```python
from build123d import *

# Parameters (mm, degrees)
F1_DEPTH  = 60
F3_DEPTH  = 10
F5_DEPTH  = 10
F6_R      = 1.5
F7_R      = 1.5
F8_R      = 1.5
F9_R      = 1.5
F10_DEPTH = 10
F11_R     = 3.5
F12_DEPTH = 4
F13_R     = 1.5
F14_DEPTH = 6


# Not quite as in the source:
# - a feature names something its author has since deleted; it is built from what else it names


with BuildPart() as f1:
    # F0 (on Front) → F1 (new body)
    with BuildSketch(Plane.XZ):
        Polygon((-40, 60), (-40, 0), (40, 0), (40, 60), (30, 60), (30, 20), (12, 20), (12, 10), (-12, 10), (-12, 20), (-30, 20), (-30, 60), align=None)
    extrude(amount=F1_DEPTH)

    # F2 (on face) → F3 (cut, through all)
    with BuildSketch(Plane.YZ.offset(40)):
        with BuildLine():
            ThreePointArc((-33.5355339059, 48.5355339059), (-30, 47.0710678119), (-26.4644660941, 48.5355339059))
            Line((-26.4644660941, 48.5355339059), (-15, 60))
            Line((-15, 60), (-45, 60))
            Line((-45, 60), (-33.5355339059, 48.5355339059))
        make_face()
    extrude(amount=-F3_DEPTH, mode=Mode.SUBTRACT)

    # F4 (on face) → F5 (cut, through all)
    with BuildSketch(Plane(origin=(-40, 0, 0), x_dir=(0, -1, 0), z_dir=(-1, 0, 0))):
        with BuildLine():
            Line((37.5, 60), (22.5, 60))
            Line((22.5, 60), (26.4644660941, 56.0355339059))
            ThreePointArc((26.4644660941, 56.0355339059), (30, 54.5710678119), (33.5355339059, 56.0355339059))
            Line((33.5355339059, 56.0355339059), (37.5, 60))
        make_face()
    extrude(amount=-F5_DEPTH, mode=Mode.SUBTRACT)

    # F6 (on face) + F7 (on face) + F8 (on face) + F9 (on face) → F10 (cut)
    with BuildSketch(Plane.XY.offset(60)):
        with Locations((-35, -7.5)):
            Circle(F6_R)
    with BuildSketch(Plane.XY.offset(60)):
        with Locations((-35, -52.5)):
            Circle(F7_R)
    with BuildSketch(Plane.XY.offset(60)):
        with Locations((35, -7.5)):
            Circle(F8_R)
    with BuildSketch(Plane.XY.offset(60)):
        with Locations((35, -52.5)):
            Circle(F9_R)
    extrude(amount=-F10_DEPTH, mode=Mode.SUBTRACT)

    # F11 (on face) → F12 (cut)
    with BuildSketch(Plane(origin=(0, 0, 0), x_dir=(1, 0, 0), z_dir=(0, 0, -1))):
        with Locations((0, 30)):
            Circle(F11_R)
    extrude(amount=-F12_DEPTH, mode=Mode.SUBTRACT)

    # F13 (on face) → F14 (cut, through all)
    with BuildSketch(Plane(origin=(0, 0, 4), x_dir=(1, 0, 0), z_dir=(0, 0, -1))):
        with Locations((0, 30)):
            Circle(F13_R)
    extrude(amount=-F14_DEPTH, mode=Mode.SUBTRACT)


solid = f1.part
```
Input: part model. Units: mm. Frame: model coordinates. A direction names the side the tool comes from. Coordinates: 2 decimals unless noted, no trailing zeros. Loops run counter-clockwise (first coordinate to the right, second up) from the corner with the lowest first, then second, coordinate; pieces in that order, holes last. Notation, with made-up numbers: (14, -4.75) - (30, -4.75) arc R24 cw to (30, 33.25) - close; hole circle Ø1 at (-33.5, 29.25). An arc over 180 degrees is marked (long way). Answer in a Markdown table with one row per item.
(1) Mould query, pull axis Y, two halves, no side actions, for faces 5 (the face through (2, -30, 4)), 6 (the face through (-1, 0, 4)), 7 (the face through (21, -30, 20)), 8 (the face through (-35.07, -29.95, 54.57)). Classes: pulls with the +Y half, pulls with the -Y half, needs draft (parallel to the pull), parting line crosses it, or undercut.
Model answer:
| item | result |
|---|---|
| face 5 | undercut |
| face 6 | pulls with the +Y half |
| face 7 | needs draft |
| face 8 | undercut |
(2) Cut plane C-C on y = -30. Output: boundary loops of the cut face in (x, z), plus the area to 3 significant figures.
Model answer:
| item | result |
|---|---|
| outline | (-40, 0) - (-3.5, 0) - (-3.5, 4) - (-1.5, 4) - (-1.5, 10) - (-12, 10) - (-12, 20) - (-30, 20) - (-30, 54.57) - (-40, 54.57) - close; (1.5, 4) - (3.5, 4) - (3.5, 0) - (40, 0) - (40, 47.07) - (30, 47.07) - (30, 20) - (12, 20) - (12, 10) - (1.5, 10) - close |
| area | 1,930 mm² |
(3) Material intervals for L1, parallel to X at y = -30, z = 2.8; L2, parallel to X at y = -19, z = 14.5; L3, parallel to Y at x = -35, z = 55.5, sorted ascending. Write a range as from..to.
Model answer:
| item | result |
|---|---|
| L1 | x = -40..-3.5, 3.5..40 |
| L2 | x = -40..-12, 12..40 |
| L3 | y = -60..-54, -51..-32.9, -27.1..-9, -6..0 |
(4) Set-up query: faces 1 (the face through (12, -30, 15)), 2 (the face through (-35.1, -35.5, 58)), 3 (the face through (35, -7, 50)), 4 (the face through (35, -21, 54)). Return all of +Z, -Z, +X, -X, +Y, -Y with unobstructed straight access to the full face (end or side cutting, diameter ignored); none if empty.
Model answer:
| item | result |
|---|---|
| face 1 | +Z, +Y, -Y |
| face 2 | +Z, +X, -X |
| face 3 | +Z |
| face 4 | +Z, +X |
(5) Pin query (flat end, axial travel): P1, Ø5, axis at x = 0, y = -30, coming from the +Z side; P2, Ø0.9, axis at x = -34.5, y = -8, coming from the +Z side; P3, Ø20, axis at x = -19, y = -24, coming from the +Z side. Return the tip coordinate at first contact, or that it passes through.
Model answer:
| item | result |
|---|---|
| P1 | stops at z = 10 |
| P2 | stops at z = 50 |
| P3 | stops at z = 20 |
(6) Cut plane A-A on x = 0. Output: boundary loops of the cut face in (y, z), plus the area to 3 significant figures.
Model answer:
| item | result |
|---|---|
| outline | (-60, 0) - (-33.5, 0) - (-33.5, 4) - (-31.5, 4) - (-31.5, 10) - (-60, 10) - close; (-28.5, 4) - (-26.5, 4) - (-26.5, 0) - (0, 0) - (0, 10) - (-28.5, 10) - close |
| area | 554 mm² |
(7) Cut plane B-B on z = 11. Output: boundary loops of the cut face in (x, y).
Model answer:
| item | result |
|---|---|
| outline | (-40, -60) - (-12, -60) - (-12, 0) - (-40, 0) - close; (12, -60) - (40, -60) - (40, 0) - (12, 0) - close |
(8) Cut plane D-D on y = -4.5. Output: boundary loops of the cut face in (x, z), plus the area to 3 significant figures.
Model answer:
| item | result |
|---|---|
| outline | (-40, 0) - (40, 0) - (40, 60) - (30, 60) - (30, 20) - (12, 20) - (12, 10) - (-12, 10) - (-12, 20) - (-30, 20) - (-30, 60) - (-40, 60) - close |
| area | 2,160 mm² |
